```python
from build123d import *

# Parameters (mm, degrees)
BOSS_EXTRUDE1_DEPTH = 4
SKETCH2_R           = 2
SKETCH2_R_2         = 1.5
CUT_EXTRUDE1_DEPTH  = 20
SKETCH3_R           = 1.5
CUT_EXTRUDE2_DEPTH  = 10
SKETCH5_R           = 1.5
SKETCH5_R_2         = 2
CUT_EXTRUDE3_DEPTH  = 5
SKETCH7_R           = 1.5
CUT_EXTRUDE4_DEPTH  = 10


with BuildPart() as part:
    # Sketch1 → Boss-Extrude1 (new body)
    with BuildSketch(Plane.XY):
        with BuildLine():
            Line((-95, -115), (-95, -195))
            ThreePointArc((-95, -195), (-93.535533906, -198.535533906), (-90, -200))
            Line((-90, -200), (90, -200))
            ThreePointArc((90, -200), (93.535533906, -198.535533906), (95, -195))
            Line((95, -195), (95, -117.93976744))
            ThreePointArc((95, -117.93976744), (93.535533906, -114.404233535), (90, -112.93976744))
            Line((90, -112.93976744), (60, -112.93976744))
            ThreePointArc((60, -112.93976744), (56.464466094, -111.475301346), (55, -107.93976744))
            Line((55, -107.93976744), (55, -47.93976744))
            ThreePointArc((55, -47.93976744), (56.464466094, -44.404233535), (60, -42.93976744))
            Line((60, -42.93976744), (90, -42.93976744))
            ThreePointArc((90, -42.93976744), (93.535533906, -41.475301346), (95, -37.93976744))
            Line((95, -37.93976744), (95, -5))
            ThreePointArc((95, -5), (93.535533906, -1.464466094), (90, 0))
            Line((90, 0), (-90, 0))
            ThreePointArc((-90, 0), (-93.535533906, -1.464466094), (-95, -5))
            Line((-95, -5), (-95, -35))
            ThreePointArc((-95, -35), (-93.535533906, -38.535533906), (-90, -40))
            Line((-90, -40), (-60, -40))
            ThreePointArc((-60, -40), (-56.464466094, -41.464466094), (-55, -45))
            Line((-55, -45), (-55, -105))
            ThreePointArc((-55, -105), (-56.464466094, -108.535533906), (-60, -110))
            Line((-60, -110), (-90, -110))
            ThreePointArc((-90, -110), (-93.535533906, -111.464466094), (-95, -115))
        make_face()
    extrude(amount=BOSS_EXTRUDE1_DEPTH)

    # Sketch2 → Cut-Extrude1 (cut)
    with BuildSketch(Plane.XY.offset(4)):
        with Locations((-85, -185)):
            Circle(SKETCH2_R)
        with Locations((-85, -15)):
            Circle(SKETCH2_R)
        with Locations((85, -15)):
            Circle(SKETCH2_R)
        with Locations((85, -185)):
            Circle(SKETCH2_R)
        with Locations((-6.765, -180)):
            Circle(SKETCH2_R_2)
        with Locations((6.765, -180)):
            Circle(SKETCH2_R_2)
    extrude(amount=-CUT_EXTRUDE1_DEPTH, mode=Mode.SUBTRACT)

    # Sketch3 → Cut-Extrude2 (cut)
    with BuildSketch(Plane.XY.offset(4)):
        with Locations((-71.25, -25)):
            Circle(SKETCH3_R)
        with Locations((-71.25, -75)):
            Circle(SKETCH3_R)
        with Locations((-71.25, -175)):
            Circle(SKETCH3_R)
        with Locations((-71.25, -125)):
            Circle(SKETCH3_R)
        with Locations((71.25, -125)):
            Circle(SKETCH3_R)
        with Locations((71.25, -75)):
            Circle(SKETCH3_R)
        with Locations((71.25, -25)):
            Circle(SKETCH3_R)
        with Locations((-23.75, -125)):
            Circle(SKETCH3_R)
        with Locations((-23.75, -175)):
            Circle(SKETCH3_R)
        with Locations((-47.5, -125)):
            Circle(SKETCH3_R)
        with Locations((-47.5, -175)):
            Circle(SKETCH3_R)
    extrude(amount=-CUT_EXTRUDE2_DEPTH, mode=Mode.SUBTRACT)

    # Sketch5 → Cut-Extrude3 (cut, through all)
    with BuildSketch(Plane.XY.offset(4)):
        with Locations((-40, -60)):
            Circle(SKETCH5_R)
        with Locations((-40, -80)):
            Circle(SKETCH5_R)
        with Locations((40, -80)):
            Circle(SKETCH5_R)
        with Locations((40, -60)):
            Circle(SKETCH5_R)
        with Locations((20.1, -132.9)):
            Circle(SKETCH5_R)
        with Locations((15, -185)):
            Circle(SKETCH5_R)
        with Locations((63.2, -183.7)):
            Circle(SKETCH5_R)
        with Locations((48, -132.9)):
            Circle(SKETCH5_R)
        with Locations((0, -7)):
            Circle(SKETCH5_R_2)
        with Locations((0, -40)):
            Circle(SKETCH5_R_2)
        with Locations((-37, -23.5)):
            Circle(SKETCH5_R)
        with Locations((37, -23.5)):
            Circle(SKETCH5_R)
    extrude(amount=-CUT_EXTRUDE3_DEPTH, mode=Mode.SUBTRACT)

    # Sketch7 → Cut-Extrude4 (cut)
    with BuildSketch(Plane(origin=(0, 0, 0), x_dir=(-1, 0, 0), z_dir=(0, 0, -1))):
        with Locations((12.568709429, -57.035989116)):
            Circle(SKETCH7_R)
        with Locations((12.5, -68.035774524)):
            Circle(SKETCH7_R)
        with Locations((-12.5, -68.035774524)):
            Circle(SKETCH7_R)
        with Locations((-12.568709429, -57.035989116)):
            Circle(SKETCH7_R)
        with BuildLine():
            Line((17, -110), (-17, -110))
            ThreePointArc((-17, -110), (-19.121320344, -109.121320344), (-20, -107))
            Line((-20, -107), (-20, -98))
            ThreePointArc((-20, -98), (-19.121320344, -95.878679656), (-17, -95))
            Line((-17, -95), (17, -95))
            ThreePointArc((17, -95), (19.121320344, -95.878679656), (20, -98))
            Line((20, -98), (20, -107))
            ThreePointArc((20, -107), (19.121320344, -109.121320344), (17, -110))
        make_face()
    extrude(amount=-CUT_EXTRUDE4_DEPTH, mode=Mode.SUBTRACT)


solid = part.part
```
Geometry check sheet. Reference: the model listing, model coordinates, mm. A direction names the side the tool comes from. Round coordinates to 2 decimals unless told otherwise and drop trailing zeros. Order: outer loops, then holes, each group sorted by start corner. A loop starts at its lowest first (then second) coordinate and runs counter-clockwise, first axis right, second up. Notation, with made-up numbers: (68, 71.5) - (82, 71.5) arc R25 cw to (82, 89.5) - close; hole circle Ø3 at (10, -34). An arc over 180 degrees is marked (long way). Use a Markdown table: item, result. Add a question column.
(1) Tool access check on faces 1 (the cylindrical face through (93.57, -114.44, 1.97)), 2 (the cylindrical face through (-94, -38, 2)), 3 (the cylindrical face through (-93, -1, 2)). Record the directions out of +Z, -Z, +X, -X, +Y, -Y that give a thin tool (end or side, any length) a straight path to the whole face; none if there is none.
(2) Material ranges on line 1 along Y through (x, z) = (63, 1.2); line 2 along Y through (x, z) = (40, 2.65); line 3 along Y through (x, z) = (-71.25, 3), recorded low to high. Write a range as [from, to].
(3) Depth check by flat-ended pin: pin 1 (3.5 mm diameter, centred on x = 37, y = -23.5, fed in from -Z); pin 2 (3.5 mm diameter, centred on x = 0, y = -7, fed in from -Z); pin 3 (2 mm diameter, centred on y = -101, z = 2.5, fed in from -X). Enter the tip coordinate at first touch or a pass-through.
(4) Sectioned sample at B-B, the plane z = 1.7. Count the separate pieces of the cut face and the enclosed holes in it, and give its area (3 significant figures).
(5) Release check for a two-part mould opening along Y. For faces 4 (the flat face through (-1, -121, 0)), 5 (the cylindrical face through (-56, -108, 2)), 6 (the cylindrical face through (-93, -111, 2)), 7 (the cylindrical face through (94, -2, 2)) record: pulls with the +Y half, pulls with the -Y half, needs draft (parallel to the pull), parting line crosses it, or undercut.
(6) Sectioned sample at A-A, the plane x = 76. Enter the section's corners in (y, z).
Answers below:
| question | item | result |
|---|---|---|
| 1 | face 1 | +Z, -Z, +X |
| 1 | face 2 | +Z, -Z, -X |
| 1 | face 3 | +Z, -Z, -X, +Y |
| 2 | line 1 | [-200, -185.19], [-182.21, -112.94], [-42.94, 0] |
| 2 | line 2 | [-200, -81.5], [-78.5, -61.5], [-58.5, 0] |
| 2 | line 3 | [-200, -176.5], [-173.5, -126.5], [-123.5, -110], [-40, -26.5], [-23.5, 0] |
| 3 | pin 1 | z = 0 |
| 3 | pin 2 | through |
| 3 | pin 3 | x = -55 |
| 4 | separate pieces | 1 |
| 4 | enclosed holes | 32 |
| 4 | area | 31,500 mm² |
| 5 | face 4 | needs draft |
| 5 | face 5 | undercut |
| 5 | face 6 | undercut |
| 5 | face 7 | pulls with the +Y half |
| 6 | outline | (-200, 0) - (-112.94, 0) - (-112.94, 4) - (-200, 4) - close; (-42.94, 0) - (0, 0) - (0, 4) - (-42.94, 4) - close |
